Part print with two shaded views. Sizes in mm from the minimum x, y, z corner. Coordinates: 2 decimals unless noted, no trailing zeros. Write each loop counter-clockwise with the first axis right and the second up, starting at its lowest first coordinate (ties: lowest second). Pieces come first, ordered by that corner, then holes. Notation, with made-up numbers: (56.25, 68.25) - (65.25, 68.25) arc R16 cw to (65.25, 79.25) - close; hole circle Ø7 at (-26.75, 1.25). An arc over 180 degrees is marked (long way). One line per question, with ' | ' between items. Start each with the question number.
1. Band-saw the part on B-B, the plane x = 66. Write the cut outline in (y, z).
2. Band-saw the part on C-C, the plane x = 84. Write the cut outline in (y, z), then the cut area to 3 significant figures.
3. Probe line 1 (Y direction, x = 52.5, z = 1.45); line 2 (Y direction, x = 78, z = 1.9). List the from-to ranges inside material, lowest first.
4. Band-saw the part on A-A, the plane z = 0.55. Write the cut outline in (x, y), then the cut area to 3 significant figures.
5. Flat gauge pins, fed straight in: P1, Ø1.5, axis at y = 129, z = 2, coming from the -X side; P2, Ø1.5, axis at x = 43, z = 1, coming from the +Y side; P3, Ø1.5, axis at x = 51.5, z = 2, coming from the -Y side. Where does each tip first touch, or does it go through?
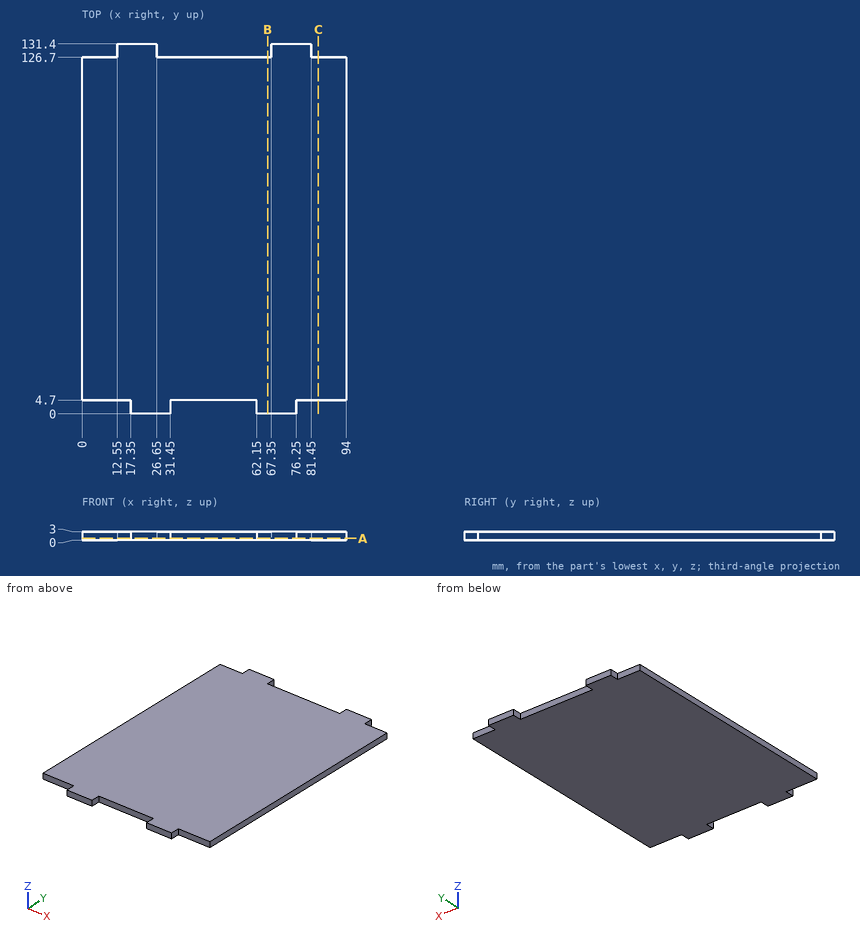
Filled in:
1) outline: (0, 0) - (126.7, 0) - (126.7, 3) - (0, 3) - close
2) outline: (4.7, 0) - (126.7, 0) - (126.7, 3) - (4.7, 3) - close | area: 366 mm²
3) line 1: y = 4.7 to 126.7 | line 2: y = 4.7 to 131.4
4) outline: (0, 4.7) - (17.35, 4.7) - (17.35, 0) - (31.45, 0) - (31.45, 4.7) - (62.15, 4.7) - (62.15, 0) - (76.25, 0) - (76.25, 4.7) - (94, 4.7) - (94, 126.7) - (81.45, 126.7) - (81.45, 131.4) - (67.35, 131.4) - (67.35, 126.7) - (26.65, 126.7) - (26.65, 131.4) - (12.55, 131.4) - (12.55, 126.7) - (0, 126.7) - close | area: 11,700 mm²
5) P1: stops at x = 12.55 | P2: stops at y = 126.7 | P3: stops at y = 4.7
